from build123d import *

# Parameters (mm, degrees)
F0_W     = 152.4
F0_H     = 152.4
F1_DEPTH = 50.8
F3_DEPTH = 152.401
F5_DEPTH = 7.62
F7_DEPTH = 7.62
F9_DEPTH = 167.64


with BuildPart() as f1:
    # F0 (on Top) → F1 (new body)
    with BuildSketch(Plane.XY):
        Rectangle(F0_W, F0_H)
    extrude(amount=F1_DEPTH)

    # F2 (on face) → F3 (cut, through all)
    with BuildSketch(Plane(origin=(-76.2, 0, 0), x_dir=(0, -1, 0), z_dir=(-1, 0, 0))):
        Polygon((76.2, 50.8), (0, 50.8), (76.2, 0), align=None)
        Polygon((-76.2, 0), (0, 50.8), (-76.2, 50.8), align=None)
    extrude(amount=-F3_DEPTH, mode=Mode.SUBTRACT)

    # F4 (on face) → F5 (join)
    with BuildSketch(Plane.YZ.offset(76.2)):
        Polygon((-76.2, 0), (-73.66, 0), (0, 49.1066666667), (73.66, 0), (76.2, 0), (0, 50.8), align=None)
    extrude(amount=F5_DEPTH)

    # F6 (on face) → F7 (join)
    with BuildSketch(Plane(origin=(-76.2, 0, 0), x_dir=(0, -1, 0), z_dir=(-1, 0, 0))):
        Polygon((-76.2, 0), (-73.66, 0), (0, 49.0982), (73.66, 0), (76.2, 0), (0, 50.8), align=None)
    extrude(amount=F7_DEPTH)

    # F8 (on face) → F9 (join)
    with BuildSketch(Plane.YZ.offset(83.82)):
        Polygon((-86.3404464857, -8.4536309905), (-73.66, 0), (-76.2, 0), (-88.8804464857, -8.4536309905), align=None)
        Polygon((76.2, 0), (73.66, 0), (86.3404464857, -8.4536309905), (88.8804464857, -8.4536309905), align=None)
    extrude(amount=-F9_DEPTH)


solid = f1.part
Can you work these out from the model? Positions are in its coordinate system, mm. A direction names the side the tool comes from. Give positions to 0.01 mm unless a question says otherwise; leave off trailing zeros. Write each loop counter-clockwise with the first axis right and the second up, starting at its lowest first coordinate (ties: lowest second). Pieces come first, ordered by that corner, then holes. Notation, with made-up numbers: (54, -6) -> (92, -6) arc R20 ccw to (92, 24) -> close; hole circle Ø8 at (69.5, 77). An arc over 180 degrees is marked (long way). Answer as a JSON object with one key per item and string values. Group by question number.
Item 1: Please list where these lines run through material, in increasing order: line 1 (X direction, y = 32, z = 19); line 2 (Y direction, x = -56, z = -4.5); line 3 (Y direction, x = -19.5, z = -3). Write a range as [from, to].
Item 2: Suppose I cut it at C-C (y = -14). Please give me the cut outline in (x, z), plus the area to 3 significant figures.
Item 3: Suppose I cut it at B-B (x = -39.5). Please give me the cut outline in (y, z), plus the area to 3 significant figures.
Item 4: I'm going to push flat-ended pins straight in: P1, Ø8, axis at x = 56, z = 6, coming from the +Y side; P2, Ø4, axis at x = -45, y = 62, coming from the -Z side; P3, Ø1.5, axis at x = 60, y = 17.5, coming from the +Z side. Where does each tip first touch, or does it pass through?
Item 5: Suppose I cut it at A-A (z = -5). Please give me the cut outline in (x, y).
Item 6: Suppose I cut it at D-D (z = 20). Please give me the cut outline in (x, y).
Item 7: For faces 4 (the face through (1, 1, 0)), 5 (the face through (-83.82, 13, 41)), which set-ups out of +Z, -Z, +X, -X, +Y, -Y let a thin tool reach every point of the face, with its end or its side?
Item 8: We'd pull the mould along Y, two halves only. Please class faces 1 (the face through (-76.2, -1, 19)), 2 (the face through (76.2, -1, 19)), 3 (the face through (83.82, 13, 41)): +Y half, -Y half, draft (parallel to the pull), parting line (faces both ways), or undercut.
Findings:
{
 "1": {"line 1": "x = [-76.2, 76.2]", "line 2": "y = [-82.95, -80.41], [80.41, 82.95]", "line 3": "y = [-80.7, -78.16], [78.16, 80.7]"},
 "2": {"outline": "(-83.82, 39.77) -> (-76.2, 39.77) -> (-76.2, 0) -> (76.2, 0) -> (76.2, 39.77) -> (83.82, 39.77) -> (83.82, 41.47) -> (-83.82, 41.47) -> close", "area": "6,350 mm²"},
 "3": {"outline": "(-88.88, -8.45) -> (-86.34, -8.45) -> (-73.66, 0) -> (73.66, 0) -> (86.34, -8.45) -> (88.88, -8.45) -> (0, 50.8) -> close", "area": "3,910 mm²"},
 "4": {"P1": "stops at y = 73.2", "P2": "stops at z = 0", "P3": "stops at z = 39.63"},
 "5": {"outline": "(-83.82, -83.7) -> (83.82, -83.7) -> (83.82, -81.16) -> (-83.82, -81.16) -> close; (-83.82, 81.16) -> (83.82, 81.16) -> (83.82, 83.7) -> (-83.82, 83.7) -> close"},
 "6": {"outline": "(-83.82, -46.2) -> (83.82, -46.2) -> (83.82, -43.66) -> (76.2, -43.66) -> (76.2, 43.66) -> (83.82, 43.66) -> (83.82, 46.2) -> (-83.82, 46.2) -> (-83.82, 43.65) -> (-76.2, 43.65) -> (-76.2, -43.65) -> (-83.82, -43.65) -> close"},
 "7": {"face 4": "-Z, +X, -X", "face 5": "+Z, -Z, -X, +Y, -Y"},
 "8": {"face 1": "undercut", "face 2": "undercut", "face 3": "draft"}
}
